Geometry: final body of the model. Coordinates: model frame, mm. A direction names the side the tool comes from. Coordinates: 2 decimals unless noted, no trailing zeros. Write each loop counter-clockwise with the first axis right and the second up, starting at its lowest first coordinate (ties: lowest second). Pieces come first, ordered by that corner, then holes. Notation, with made-up numbers: M -5.5,35.5 L 33.5,35.5 A23 ccw 33.5,49.5 Z; hole C 85.25,60 d3. An arc over 180 degrees is marked long. Write item = value, one per line. Start each with the question number.
Item 1: Ray query, L1, parallel to X at y = 0.45, z = 7; L2, parallel to Y at x = 0.4, z = 4.75; L3, parallel to Z at x = -0.9, y = -0.1. Return the intervals inside material, ascending. Write a range as [from, to].
Item 2: Pull-direction query (X, two-part tool) for faces 3 (the flat face through (0, 0, 0)), 4 (the flat face through (0, 0.951, 6)), 5 (the conical face through (2.024, 0.637, 6.207)); classes: +X half, -X half, draft (parallel to the pull), parting line (faces both ways), or undercut.
Item 3: Section B-B on z = 1.5. Output: boundary loops of the cut face in (x, y), plus the area to 3 significant figures.
Item 4: Section A-A on z = 6.25. Output: boundary loops of the cut face in (x, y).
Item 5: Reachability of faces 1 (the flat face through (-0.948, 0, 6)), 2 (the cylindrical face through (-0.54, -2.44, 0.85)) from +Z, -Z, +X, -X, +Y, -Y: full face, straight path, thin tool, end or side. Return the list, or none.
Item 6: First-contact query: pin 1 Ø1 at (y, z) = (2, 7) entering from +X; pin 2 Ø2 at (y, z) = (0.5, 7) entering from +X; pin 3 Ø2 at (x, z) = (-0.5, 7) entering from +Y. Flat tips, straight axial feed; report the tip coordinate or a pass-through.
from build123d import *

# Parameters (mm, degrees)
SKETCH_1_R          = 2.5
EXTRUDE_1_DEPTH     = 1.7
FILLET_7_R          = 0.5
SKETCH_7_R          = 2.050609665
SKETCH_8_R          = 2.2
SKETCH_10_W         = 1.896668422
SKETCH_10_H         = 1.902308834
CUT_EXTRUDE_1_DEPTH = 4
FILLET_13_R         = 0.5
FILLET_17_R         = 2
FILLET_18_R         = 0.5
FILLET_19_R         = 0.5


with BuildPart() as part:
    # 草图1 → 凸台-拉伸1 (new body)
    with BuildSketch(Plane.XY):
        Circle(SKETCH_1_R)
    extrude(amount=EXTRUDE_1_DEPTH)

    # 圆角7
    fillet_7_edges = [part.edges().sort_by_distance(p)[0] for p in [
        (-2.5, 0, 0),
    ]]
    fillet(fillet_7_edges, radius=FILLET_7_R)

    # 放样1: read off the stored shape, not the designer's step
    # 放样1: loft between two sections, ruled curve by curve
    loft_1_from = [
        Edge.make_bspline([(0.665743614, 0.998391427, 1.7), (-1.33103924, 2.329878654, 1.7), (-2.662526467, 0.333095801, 1.7), (-0.665743614, -0.998391427, 1.7), (1.33103924, -2.329878654, 1.7), (2.662526467, -0.333095801, 1.7), (0.665743614, 0.998391427, 1.7)], [0, 0, 0, 0, 0.5, 0.5, 0.5, 1, 1, 1, 1], 3, [1, 0.333333333, 0.333333333, 1, 0.333333333, 0.333333333, 1]),
    ]
    loft_1_to = [
        Edge.make_bspline([(1.45, 1.45, 4.3), (-1.45, 4.35, 4.3), (-4.35, 1.45, 4.3), (-1.45, -1.45, 4.3), (1.45, -4.35, 4.3), (4.35, -1.45, 4.3), (1.45, 1.45, 4.3)], [0, 0, 0, 0, 0.5, 0.5, 0.5, 1, 1, 1, 1], 3, [1, 0.333333333, 0.333333333, 1, 0.333333333, 0.333333333, 1]),
    ]
    loft_1 = Solid(Shell([*[Face.make_surface_from_curves(loft_1_from[k], loft_1_to[k]) for k in range(1)], Face(Wire(loft_1_from)), Face(Wire(loft_1_to))]))
    add(loft_1)

    # 草图7 → 放样3 section 0
    with BuildSketch(Plane.XY.offset(4.3)):
        Circle(SKETCH_7_R)
    # 草图8 → 放样3 section 1
    with BuildSketch(Plane.XY.offset(8.3)):
        Circle(SKETCH_8_R)
    loft()

    # 草图10 → 切除-拉伸1 (cut)
    with BuildSketch(Plane.XY.offset(8.3)):
        Rectangle(SKETCH_10_W, SKETCH_10_H)
    extrude(amount=-CUT_EXTRUDE_1_DEPTH, mode=Mode.SUBTRACT)

    # 圆角13
    fillet_13_edges = [part.edges().sort_by_distance(p)[0] for p in [
        (-2.5, 0, 1.7),
    ]]
    fillet(fillet_13_edges, radius=FILLET_13_R)

    # 圆角17
    fillet_17_edges = [part.edges().sort_by_distance(p)[0] for p in [
        (-1.894516299, -0.784734346, 4.3),
    ]]
    fillet(fillet_17_edges, radius=FILLET_17_R)

    # 圆角18
    fillet_18_edges = [part.edges().sort_by_distance(p)[0] for p in [
        (-0.665743614, -0.998391427, 1.7),
    ]]
    fillet(fillet_18_edges, radius=FILLET_18_R)

    # 圆角19
    fillet_19_edges = [part.edges().sort_by_distance(p)[0] for p in [
        (-2.2, 0, 8.3),
    ]]
    fillet(fillet_19_edges, radius=FILLET_19_R)


solid = part.part
Responses:
q1.L1 = [-2.1, -0.95], [0.95, 2.1]
q1.L2 = [-2.03, -0.95], [0.95, 2.03]
q1.L3 = [0, 4.3]
q2.face_3 = draft
q2.face_4 = undercut
q2.face_5 = parting line
q3.outline = C 0,0 d4.8
q3.area = 18.1 mm²
q4.outline = C 0,0 d4.25; hole M -0.95,-0.95 L 0.95,-0.95 L 0.95,0.95 L -0.95,0.95 Z
q5.face_1 = +Z
q5.face_2 = +Z, -Z
q6.pin_1 = 1.54
q6.pin_2 = 2.18
q6.pin_3 = 2.18
